from build123d import *

# Parameters (mm, degrees)
HORN_START                = 52.8
HORN_DOG_POCKET_DEPTH     = 4.2
HUB_START                 = 52.8
SKETCH3_R                 = 8
HUB_RELIEF_DEPTH          = 1.7
CENTRE_START              = 52.8
SKETCH4_R                 = 4
CENTRE_CABLE_KIDNEY_DEPTH = 6.4
TOWER_START               = 52.8
SKETCH5_R                 = 1.7
TOWER_BOLT_HOLES_DEPTH    = 6.4
TOWER_NUT_POCKETS_DEPTH   = 2.9


with BuildPart() as part:
    # Sketch1 → Turntable (revolve)
    with BuildSketch(Plane.XY, mode=Mode.PRIVATE) as turntable_sk:
        Polygon((0, 53), (70, 53), (70, 55), (66, 59), (0, 59), align=None)
    revolve(turntable_sk.sketch.rotate(Axis((0, 40, 0), (0, 1, 0)), 90), axis=Axis((0, 40, 0), (0, 1, 0)))

    # Sketch2 → Horn dog pocket (cut)
    with BuildSketch(Plane(origin=(0, 0, 0), x_dir=(1, 0, 0), z_dir=(0, 1, 0)).offset(HORN_START)):
        with BuildLine():
            Line((-23.1, -4.4), (23.1, -4.4))
            ThreePointArc((23.1, -4.4), (27.5, 0), (23.1, 4.4))
            Line((23.1, 4.4), (-23.1, 4.4))
            ThreePointArc((-23.1, 4.4), (-27.5, 0), (-23.1, -4.4))
        make_face()
    extrude(amount=HORN_DOG_POCKET_DEPTH, mode=Mode.SUBTRACT)

    # Sketch3 → Hub relief (cut)
    with BuildSketch(Plane(origin=(0, 0, 0), x_dir=(1, 0, 0), z_dir=(0, 1, 0)).offset(HUB_START)):
        Circle(SKETCH3_R)
    extrude(amount=HUB_RELIEF_DEPTH, mode=Mode.SUBTRACT)

    # Sketch4 → Centre + cable kidney (cut)
    with BuildSketch(Plane(origin=(0, 0, 0), x_dir=(1, 0, 0), z_dir=(0, 1, 0)).offset(CENTRE_START)):
        with Locations(Location((0, 0, 0), (0, 0, 270))):
            Circle(SKETCH4_R)
        with BuildLine():
            ThreePointArc((-35.238044383, 29.568230046), (0, 46), (35.238044383, 29.568230046))
            ThreePointArc((35.238044383, 29.568230046), (34.498503383, 21.115237729), (26.045511066, 21.854778729))
            ThreePointArc((26.045511066, 21.854778729), (0, 34), (-26.045511066, 21.854778729))
            ThreePointArc((-26.045511066, 21.854778729), (-34.498503383, 21.115237729), (-35.238044383, 29.568230046))
        make_face()
    extrude(amount=CENTRE_CABLE_KIDNEY_DEPTH, mode=Mode.SUBTRACT)

    # Sketch5 → Tower bolt holes (cut)
    with BuildSketch(Plane(origin=(0, 0, 0), x_dir=(1, 0, 0), z_dir=(0, 1, 0)).offset(TOWER_START)):
        with Locations(Location((-26, 44, 0), (0, 0, 90))):
            Circle(SKETCH5_R)
        with Locations(Location((-26, -22, 0), (0, 0, 90))):
            Circle(SKETCH5_R)
        with Locations(Location((26, 44, 0), (0, 0, 90))):
            Circle(SKETCH5_R)
        with Locations(Location((26, -22, 0), (0, 0, 90))):
            Circle(SKETCH5_R)
    extrude(amount=TOWER_BOLT_HOLES_DEPTH, mode=Mode.SUBTRACT)

    # Sketch6 → Tower nut pockets (cut)
    with BuildSketch(Plane(origin=(0, 0, 0), x_dir=(1, 0, 0), z_dir=(0, 1, 0)).offset(TOWER_START)):
        Polygon((-23.05, 42.296816706), (-26, 40.593633412), (-28.95, 42.296816706), (-28.95, 45.703183294), (-26, 47.406366588), (-23.05, 45.703183294), align=None)
        Polygon((-23.05, -23.703183294), (-26, -25.406366588), (-28.95, -23.703183294), (-28.95, -20.296816706), (-26, -18.593633412), (-23.05, -20.296816706), align=None)
        Polygon((28.95, 42.296816706), (26, 40.593633412), (23.05, 42.296816706), (23.05, 45.703183294), (26, 47.406366588), (28.95, 45.703183294), align=None)
        Polygon((28.95, -23.703183294), (26, -25.406366588), (23.05, -23.703183294), (23.05, -20.296816706), (26, -18.593633412), (28.95, -20.296816706), align=None)
    extrude(amount=TOWER_NUT_POCKETS_DEPTH, mode=Mode.SUBTRACT)


solid = part.part
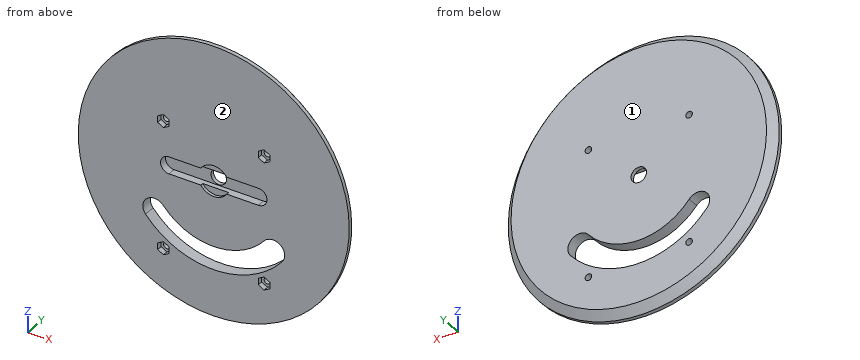
Check sheet for the modelled part. Datum: model origin and axes. Units: mm. Face numbers are marked on the shaded views. Give positions to 0.01 mm unless a question says otherwise; leave off trailing zeros. Loops run counter-clockwise (first coordinate to the right, second up) from the corner with the lowest first, then second, coordinate; pieces in that order, holes last. Notation, with made-up numbers: M -14.75,4 L 34.25,4 A28 ccw 34.25,25 Z; hole C 78,0.25 d6. An arc over 180 degrees is marked long. Answer as a JSON object with one key per item and string values. Group by question number.
Q1. Cross-section at B-B on z = -44. Give the number of separate pieces and of enclosed holes in the cut face, then the cut area to 3 significant figures.
Q2. Cross-section at A-A on z = 0. Record the cut outline in (x, y).
Q3. Go/stop test with flat-tipped pins: P1, Ø2.5, axis at x = 8, z = 0.5, coming from the -Y side; P2, Ø3, axis at x = 26.5, z = -43.5, coming from the -Y side; P3, Ø2.5, axis at x = -26, z = -44, coming from the +Y side; P4, Ø0.8, axis at y = 55, z = -44.5, coming from the +X side. Record where each tip stops, or that it passes through.
Q4. Material ranges on line 1 along X through (y, z) = (57.55, -21); line 2 along Z through (x, y) = (16.5, 56.35); line 3 along X through (y, z) = (56.95, 22), recorded low to high. Write a range as [from, to].
Q5. Release check for a two-part mould opening along Y. For the marked faces 1 and 2 record: released by +Y, released by -Y, zero draft, split by the parting line, or undercut.
Evaluation:
{
 "1": {"separate pieces": "4", "enclosed holes": "0", "area": "417 mm2"},
 "2": {"outline": "M -70,53 L -27.5,53 L -27.5,57 L -4,57 L -4,59 L -66,59 L -70,55 Z; M 4,57 L 27.5,57 L 27.5,53 L 70,53 L 70,55 L 66,59 L 4,59 Z"},
 "3": {"P1": "stops at y = 57", "P2": "stops at y = 55.7", "P3": "passes through", "P4": "stops at x = 54.36"},
 "4": {"line 1": "x = [-64.1, -34.36], [-26.93, 26.93], [34.36, 64.1]", "line 2": "z = [-66.64, -42.94], [-29.73, -4.4], [4.4, 66.64]", "line 3": "x = [-64.4, -27.7], [-24.3, 24.3], [27.7, 64.4]"},
 "5": {"face 1": "released by +Y", "face 2": "released by -Y"}
}
